Geometry check sheet. Reference: the model listing, model coordinates, mm. A direction names the side the tool comes from. Coordinates: 2 decimals unless noted, no trailing zeros. Loops run counter-clockwise (first coordinate to the right, second up) from the corner with the lowest first, then second, coordinate; pieces in that order, holes last. Notation, with made-up numbers: (-3.5, -24.75) - (39.5, -24.75) arc R28 ccw to (39.5, 4.25) - close; hole circle Ø9 at (29, 47.25). An arc over 180 degrees is marked (long way). One line per item, written item: value.
Autodesk Inventor part; units mm, degrees
ref_plane "YZ Plane" through (0, 0, 0) normal (1, 0, 0) x (0, 1, 0)
ref_plane "XZ Plane" through (0, 0, 0) normal (0, 1, 0) x (-1, 0, 0)
ref_plane "XY Plane" through (0, 0, 0) normal (0, 0, 1) x (1, 0, 0)
sketch "Sketch1" plane through (0, 0, 0) normal (0, 1, 0) x (-1, 0, 0)
  circle A0 centre (0, 0) radius 5
  circle A1 centre (0, 0) radius 1.5
  dimension "d0" = 3
  dimension "d1" = 10
extrude "Extrusion1" add sketch "Sketch1" along normal blind 4
sketch "Sketch2" plane through (0, 4, 0) normal (0, 1, 0) x (1, 0, 0)
  circle A0 centre (0, 0) radius 5
  circle A1 centre (0, 0) radius 1.5
  circle A2 centre (0, 0) radius 1.5
  circle A3 centre (0, 0) radius 4
  circle A4 centre (0, 0) radius 2.5
  dimension "d4" = 1
  dimension "d5" = 1
extrude "Extrusion2" cut sketch "Sketch2" against normal blind 0.5 contours A3
sketch "Sketch3" plane through (0, 0, 0) normal (0, -1, 0) x (1, 0, 0)
  circle A0 centre (0, 0) radius 5
  circle A1 centre (0, 0) radius 1.5
  circle A2 centre (0, 0) radius 2.5
  circle A3 centre (0, 0) radius 4
  dimension "d8" = 1
  dimension "d9" = 1
extrude "Extrusion3" cut sketch "Sketch3" against normal blind 0.5 contours A3
properties part number "bearing_d3D10b4"
(1) Cross-section at C-C on y = 2.5. Record the cut outline in (x, z), and give its area (3 significant figures).
Reply:
outline: circle Ø10 at (0, 0); hole circle Ø3 at (0, 0)
area: 71.5 mm2
(2) Cross-section at B-B on x = 0. Record the cut outline in (y, z).
Reply:
outline: (0, -5) - (4, -5) - (4, -4) - (3.5, -4) - (3.5, -2.5) - (4, -2.5) - (4, -1.5) - (0, -1.5) - (0, -2.5) - (0.5, -2.5) - (0.5, -4) - (0, -4) - close; (0, 1.5) - (4, 1.5) - (4, 2.5) - (3.5, 2.5) - (3.5, 4) - (4, 4) - (4, 5) - (0, 5) - (0, 4) - (0.5, 4) - (0.5, 2.5) - (0, 2.5) - close
(3) Cross-section at A-A on z = 0. Record the cut outline in (x, y).
Reply:
outline: (-5, 0) - (-4, 0) - (-4, 0.5) - (-2.5, 0.5) - (-2.5, 0) - (-1.5, 0) - (-1.5, 4) - (-2.5, 4) - (-2.5, 3.5) - (-4, 3.5) - (-4, 4) - (-5, 4) - close; (1.5, 0) - (2.5, 0) - (2.5, 0.5) - (4, 0.5) - (4, 0) - (5, 0) - (5, 4) - (4, 4) - (4, 3.5) - (2.5, 3.5) - (2.5, 4) - (1.5, 4) - close
(4) Material ranges on probe 1 along Z at (x, y) = (0, 3.75); probe 2 along Z at (x, y) = (0, 1.5); probe 3 along X at (y, z) = (0.95, -0.5), recorded low to high. Write a range as from..to.
Reply:
probe 1: -5..-4, -2.5..-1.5, 1.5..2.5, 4..5
probe 2: -5..-1.5, 1.5..5
probe 3: -4.97..-1.41, 1.41..4.97
(5) Access from +Z, -Z, +X, -X, +Y, -Y to the whole of each face (thin tool, end or side, straight path). Record for faces 1 (the face through (1.5, 1.97, -0.07)), 2 (the face through (-0.867, 0.246, -3.905)), 3 (the face through (2, 3.5, -2)).
Reply:
face 1: +Y, -Y
face 2: -Y
face 3: +Y
(6) Go/stop test with flat-tipped pins: pin 1 Ø1 at (y, z) = (2.5, 3.5) entering from -X; pin 2 Ø1 at (x, y) = (1.5, 2.5) entering from +Z; pin 3 Ø1.8 at (x, z) = (0, 0) entering from -Y. Record where each tip stops, or that it passes through.
Reply:
pin 1: x = -4
pin 2: z = 4.9
pin 3: through
(7) Cross-section at D-D on x = -1.75. Record the cut outline in (y, z).
Reply:
outline: (0, -4.68) - (4, -4.68) - (4, -3.6) - (3.5, -3.6) - (3.5, -1.79) - (4, -1.79) - (4, 1.79) - (3.5, 1.79) - (3.5, 3.6) - (4, 3.6) - (4, 4.68) - (0, 4.68) - (0, 3.6) - (0.5, 3.6) - (0.5, 1.79) - (0, 1.79) - (0, -1.79) - (0.5, -1.79) - (0.5, -3.6) - (0, -3.6) - close
(8) Release check for a two-part mould opening along Z. For faces 4 (the face through (-2, 4, 0)), 5 (the face through (2, 0.5, 2)), 6 (the face through (1.08, 1.97, 4.88)) record: pulls with the +Z half, pulls with the -Z half, needs draft (parallel to the pull), parting line crosses it, or undercut.
Reply:
face 4: needs draft
face 5: undercut
face 6: parting line crosses it
